from build123d import *

# Parameters (mm, degrees)
EXTRUDE_THIN1_DEPTH = 25.4
SKETCH2_R           = 3.81
CUT_EXTRUDE1_DEPTH  = 10.922
BOSS_EXTRUDE1_START = -22.225
BOSS_EXTRUDE1_DEPTH = 44.45
SKETCH4_R           = 15.875
CUT_EXTRUDE2_DEPTH  = 38.1
FILLET1_R           = 2.54


# Read off the part's stored shape, not the designer's step: Boss-Extrude1
with BuildPart() as part:
    # Sketch1 → Extrude-Thin1 (new, symmetric)
    with BuildSketch(Plane.XY):
        with BuildLine():
            Line((29.4005, 0), (16.7005, 0))
            ThreePointArc((16.7005, 0), (0, 16.7005), (-16.7005, 0))
            Line((-16.7005, 0), (-29.4005, 0))
            Line((-29.4005, 0), (-29.4005, 2.54))
            Line((-29.4005, 2.54), (-19.07210634, 2.54))
            ThreePointArc((-19.07210634, 2.54), (0, 19.2405), (19.07210634, 2.54))
            Line((19.07210634, 2.54), (29.4005, 2.54))
            Line((29.4005, 2.54), (29.4005, 0))
        make_face()
    extrude(amount=EXTRUDE_THIN1_DEPTH, both=True)

    # Sketch2 → Cut-Extrude1 (cut)
    with BuildSketch(Plane(origin=(0, 2.54, 0), x_dir=(1, 0, 0), z_dir=(0, 1, 0))):
        with Locations(Location((24.23630317, -12.7, 0), (0, 0, 270))):
            Circle(SKETCH2_R)
        with Locations(Location((24.23630317, 12.7, 0), (0, 0, 270))):
            Circle(SKETCH2_R)
        with Locations(Location((-24.27769683, 12.7, 0), (0, 0, 270))):
            Circle(SKETCH2_R)
        with Locations(Location((-24.27769683, -12.7, 0), (0, 0, 270))):
            Circle(SKETCH2_R)
    extrude(amount=-CUT_EXTRUDE1_DEPTH, mode=Mode.SUBTRACT)

    # Boss-Extrude1 outline → Boss-Extrude1 (add)
    with BuildSketch(Plane.XY.offset(BOSS_EXTRUDE1_START)):
        with BuildLine():
            ThreePointArc((6.35, 56.262443124), (0, 57.3405), (-6.35, 56.262443124))
            Line((-6.35, 56.262443124), (-6.35, 18.162443124))
            ThreePointArc((-6.35, 18.162443124), (0, 19.2405), (6.35, 18.162443124))
            Line((6.35, 18.162443124), (6.35, 56.262443124))
        make_face()
    extrude(amount=BOSS_EXTRUDE1_DEPTH)

    # Sketch4 → Cut-Extrude2 (cut)
    with BuildSketch(Plane(origin=(6.35, 0, 0), x_dir=(0, 0, -1), z_dir=(1, 0, 0))):
        with Locations((0, 37.212443124)):
            Circle(SKETCH4_R)
    extrude(amount=-CUT_EXTRUDE2_DEPTH, mode=Mode.SUBTRACT)

    # Fillet1
    fillet1_edges = [part.edges().sort_by_distance(p)[0] for p in [
        (-6.35, 18.162443124, 0),
        (0, 19.2405, 22.225),
        (6.35, 18.162443124, 0),
        (0, 19.2405, -22.225),
    ]]
    fillet(fillet1_edges, radius=FILLET1_R)


solid = part.part
CAD build for the part. Positions are in the model's coordinates, mm. A direction names the side the tool comes from. Give positions to 0.01 mm unless a question says otherwise; leave off trailing zeros. Order: outer loops, then holes, each group sorted by start corner. A loop starts at its lowest first (then second) coordinate and runs counter-clockwise, first axis right, second up. Notation, with made-up numbers: (-20.75, 85.25) -> (3.25, 85.25) arc R22 cw to (3.25, 91.25) -> close; hole circle Ø4 at (13.5, -18). An arc over 180 degrees is marked (long way). Return JSON: item names as keys, results as strings.
Q1. Which spindle directions (+Z, -Z, +X, -X, +Y, -Y) get a long thin tool onto all of the face, cutting with end or side? Do faces 1 (the face through (24, 2.54, 0)), 2 (the face through (-24, 2.54, 0)), 3 (the face through (0, 17, 25.4)). Say none if no direction does.
Working result:
{"face 1": "+Z, -Z, +X, +Y", "face 2": "+Z, -Z, -X, +Y", "face 3": "+Z, +X, -X, +Y, -Y"}
Q2. Saw through at B-B (z = 0). Write the cut outline in (x, y), then the cut area to 3 significant figures.
Working result:
{"outline": "(-29.4, 0) -> (-16.7, 0) arc R16.7 cw to (16.7, 0) -> (29.4, 0) -> (29.4, 2.54) -> (19.07, 2.54) arc R19.24 ccw to (7.85, 17.56) arc R2.54 cw to (6.35, 19.88) -> (6.35, 21.34) -> (-6.35, 21.34) -> (-6.35, 19.88) arc R2.54 cw to (-7.85, 17.56) arc R19.24 ccw to (-19.07, 2.54) -> (-29.4, 2.54) -> close; (-6.35, 53.09) -> (6.35, 53.09) -> (6.35, 56.26) arc R19.24 ccw to (-6.35, 56.26) -> close", "area": "277 mm²"}
Q3. Flat gauge pins, fed straight in: pin 1 (9 mm diameter, centred on x = -24.28, z = -12.7, fed in from +Y); pin 2 (5 mm diameter, centred on x = 19.5, z = 4, fed in from +Y); pin 3 (5 mm diameter, centred on y = 51, z = -11.5, fed in from -X). Where does each tip first touch, or does it go through?
Working result:
{"pin 1": "y = 2.54", "pin 2": "y = 9.01", "pin 3": "x = -6.35"}
Q4. Mould opens along X. For faces 4 (the face through (11.166, 15.669, 0.356)), 5 (the face through (-24.11, 1.288, 8.894)), 6 (the face through (0.09, 50.6, -8.53)), 7 (the face through (-6.77, 18.485, 0.347)) say: pulls with the +X half, pulls with the -X half, needs draft (parallel to the pull), parting line crosses it, or undercut.
Working result:
{"face 4": "parting line crosses it", "face 5": "undercut", "face 6": "needs draft", "face 7": "pulls with the -X half"}
Q5. Saw through at A-A (z = 18). Write the cut outline in (x, y), then the cut area to 3 significant figures.
Working result:
{"outline": "(-29.4, 0) -> (-16.7, 0) arc R16.7 cw to (16.7, 0) -> (29.4, 0) -> (29.4, 2.54) -> (19.07, 2.54) arc R19.24 ccw to (7.85, 17.56) arc R2.54 cw to (6.35, 19.88) -> (6.35, 56.26) arc R19.24 ccw to (-6.35, 56.26) -> (-6.35, 19.88) arc R2.54 cw to (-7.85, 17.56) arc R19.24 ccw to (-19.07, 2.54) -> (-29.4, 2.54) -> close", "area": "680 mm²"}
Q6. Saw through at C-C (y = 23). Write the cut outline in (x, z) (3 decimals).
Working result:
{"outline": "(-6.35, -22.225) -> (6.35, -22.225) -> (6.35, -7.073) -> (-6.35, -7.073) -> close; (-6.35, 7.073) -> (6.35, 7.073) -> (6.35, 22.225) -> (-6.35, 22.225) -> close"}
Q7. Drill centre lines: line 1 (X direction, y = 1.15, z = -12.7); line 2 (X direction, y = 1, z = -12); line 3 (Y direction, x = 0, z = -17). Where is each one in solid material? Low to high.
Working result:
{"line 1": "-29.4 to -28.09, -20.47 to -16.66, 16.66 to 20.43, 28.05 to 29.4", "line 2": "-29.4 to -28.02, -20.53 to -16.67, 16.67 to 20.49, 27.98 to 29.4", "line 3": "16.7 to 57.34"}
